Build history of the part. All positions in model axes, mm. A direction names the side the tool comes from. Give positions to 0.01 mm unless a question says otherwise; leave off trailing zeros. Loops run counter-clockwise (first coordinate to the right, second up) from the corner with the lowest first, then second, coordinate; pieces in that order, holes last. Notation, with made-up numbers: M 72.5,10.25 L 122.5,10.25 A23 ccw 122.5,48.25 Z; hole C 80,60 d7. An arc over 180 degrees is marked long. Put each result on its own line as item: value.
Autodesk Inventor part; units mm, degrees
ref_plane "YZ Plane" through (0, 0, 0) normal (1, 0, 0) x (0, 1, 0)
ref_plane "XZ Plane" through (0, 0, 0) normal (0, 1, 0) x (-1, 0, 0)
ref_plane "XY Plane" through (0, 0, 0) normal (0, 0, 1) x (1, 0, 0)
sketch "Sketch1" plane through (0, 0, 0) normal (0, 0, 1) x (1, 0, 0)
  circle A0 centre (0, 0) radius 40
  dimension "d0" = 80
extrude "Extrusion1" add sketch "Sketch1" along normal blind 21.5
sketch "Sketch2" plane through (0, 0, 21.5) normal (0, 0, 1) x (1, 0, 0)
  point P0 (0, 0)
  point P1 (0, 35)
  dimension "d3" = 35
hole "Hole1" at (0, 35, 21.5) direction (0, 0, -1) diameter 4.3 end through all counterbore diameter 10.59 counterbore depth 7
chamfer "Chamfer1" distance 2 distance2 3 2 edges at (-27.6179, -28.9353, 21.5) (28.9353, 27.6179, 21.5) measured on face at (-2.7418, -16.4668, 21.5)
pattern_circular "Circular Pattern1" count 6 over 360 about axis through (0, 0, 0) along (0, 0, 1) of "Hole1"
sketch "Sketch3" plane through (0, 0, 0) normal (0, 0, -1) x (-1, 0, 0)
  circle A0 centre (0, 0) radius 29.1
  dimension "d17" = 58.2
extrude "Extrusion2" cut sketch "Sketch3" against normal through all
ref_plane "Work Plane1" through (0, 0, 10.5) normal (0, 0, -1) x (-1, 0, 0)
sketch "Sketch4" plane through (0, 0, 10.5) normal (0, 0, -1) x (-1, 0, 0)
  circle A0 centre (0, 0) radius 29.5
  circle A1 centre (0, 0) radius 26.5
  dimension "d21" = 53
  dimension "d22" = 59
extrude "Extrusion3" add sketch "Sketch4" against normal blind 3
sketch "Sketch5" plane through (0, 0, 21.5) normal (0, 0, 1) x (1, 0, 0)
  arc A0 (33.6722, 21.5913) -> (1.8625, 39.9566) centre (0, 0) ccw
  line L0 (0, 0) -> (40, 0) construction
  line L1 (21.4926, 23.7527) -> (24.6091, 28.2845)
  line L2 (24.6091, 28.2845) -> (17.6054, 33.101)
  line L3 (17.6054, 33.101) -> (14.4889, 28.5691)
  line L4 (14.4889, 28.5691) -> (21.4926, 23.7527)
  line L5 (21.4926, 23.7527) -> (17.6054, 33.101) construction
  line L6 (24.6091, 28.2845) -> (14.4889, 28.5691) construction
  line L7 (17.002, 26.8409) -> (20.1185, 31.3727)
  line L8 (22.1372, 29.9845) -> (19.0207, 25.4526)
  line L9 (14.8714, 29.1253) -> (17.223, 32.5448)
  line L10 (17.223, 32.5448) -> (19.736, 30.8165)
  line L11 (19.736, 30.8165) -> (17.3845, 27.3971)
  line L12 (17.3845, 27.3971) -> (14.8714, 29.1253)
  line L13 (19.549, 28.4268) -> (16.0472, 30.8351)
  line L14 (17.3845, 27.3971) -> (17.223, 32.5448)
  line L15 (14.8714, 29.1253) -> (19.736, 30.8165)
  line L16 (0, 0) -> (17.3037, 29.9709)
  line L17 (0, 0) -> (19.549, 28.4268)
  dimension "d26" = 8.5
  dimension "d27" = 5.5
  dimension "d29" = 34.5
  dimension "d30" = 3.05
  dimension "d36" = 3
  dimension "d41" = 4.15
  dimension "d42" = 60
extrude "Extrusion4" cut sketch "Sketch5" against normal blind 1.75 contours L4 L17 L13 L7 L2 L8 | L4 L7 L13 L17 | L15 L14 L10 | L7 L13 L15 | L14 L13 L7 | L12 L16 L14 | L14 L13 L3 | L15 L3 L13 | L16 L12 L15
extrude "Extrusion7" cut sketch "Sketch5" against normal through all contours L4 L8 L2 L1
properties part number "Ring_Cover_Top"
Q1. Mould opens along X. For faces 1 (the flat face through (31, 15, 14.5)), 2 (the conical face through (39, 0, 20)), 3 (the cylindrical face through (-8.67, 39.05, 9.12)), 4 (the flat face through (-23, -19, 21.5)) say: pulls with the +X half, pulls with the -X half, needs draft (parallel to the pull), parting line crosses it, or undercut.
Here are the results:
face 1: undercut
face 2: pulls with the +X half
face 3: parting line crosses it
face 4: needs draft
Q2. Probe line 1 (Y direction, x = -26.5, z = 19); line 2 (X direction, y = -17, z = 9.5); line 3 (Y direction, x = -31, z = 12). List the from-to ranges inside material, lowest first. Write a range as from..to.
Here are the results:
line 1: -29.52..-21.18, -13.82..-12.02, 12.02..13.82, 21.18..29.52
line 2: -36.21..-32.4, -28.22..-23.62, 23.62..28.22, 32.4..36.21
line 3: -25.28..-19.54, -15.46..15.46, 19.54..25.28
Q3. Slice it at B-B (y = 0). List the corners of the cut face in (x, z).
Here are the results:
outline: M -40,0 L -29.1,0 L -29.1,10.5 L -26.5,10.5 L -26.5,13.5 L -29.1,13.5 L -29.1,21.5 L -38,21.5 L -40,18.5 Z; M 26.5,10.5 L 29.1,10.5 L 29.1,0 L 40,0 L 40,18.5 L 38,21.5 L 29.1,21.5 L 29.1,13.5 L 26.5,13.5 Z
Q4. Slice it at D-D (z = 7.25). State how many separate pieces and enclosed holes the cut face has, and give its area (3 significant figures).
Here are the results:
separate pieces: 1
enclosed holes: 8
area: 2,260 mm²
Q5. Slice it at C-C (z = 16.75). List the corners of the cut face in (x, y) (1 decimal), and give its area (3 significant figures).
Here are the results:
outline: M -35.5,-18.4 A5.3 cw long -33.7,-21.6 A40 ccw -1.9,-40 A5.3 cw long 1.9,-40 A40 ccw 33.7,-21.6 A5.3 cw long 35.5,-18.4 A40 ccw 35.5,18.4 A5.3 cw long 33.7,21.6 A40 ccw 1.9,40 A5.3 cw long -1.9,40 A40 ccw -33.7,21.6 A5.3 cw long -35.5,18.4 A40 ccw Z; hole C 0,0 d58.2; hole M 19,25.5 L 21.5,23.8 L 24.6,28.3 L 22.1,30 Z
area: 1,830 mm²
Q6. Drop flat-ended pins along their axis: pin 1 Ø5 at (y, z) = (19, 2.5) entering from +X; pin 2 Ø3 at (x, y) = (-1, 35) entering from +Z; pin 3 Ø5 at (x, z) = (-22.5, 15) entering from +Y. Give the stop position or say it passes through.
Here are the results:
pin 1: x = 36.44
pin 2: z = 14.5
pin 3: y = 34.64
Q7. Tool access for faces 5 (the flat face through (-28, 16, 14.5)), 6 (the conical face through (19.62, -33.464, 20.312)), 7 (the flat face through (23.03, 25.99, 10.9)): list every direction of +Z, -Z, +X, -X, +Y, -Y with a clear straight run to the whole face (end or side of a thin tool).
Here are the results:
face 5: +Z
face 6: +Z, +X, -Y
face 7: +Z, -Z
Q8. Slice it at A-A (x = 0). List the corners of the cut face in (y, z) (3 decimals), and give its area (3 significant figures).
Here are the results:
outline: M -40,0 L -37.15,0 L -37.15,14.5 L -40,14.5 Z; M -32.85,0 L -29.1,0 L -29.1,10.5 L -26.5,10.5 L -26.5,13.5 L -29.1,13.5 L -29.1,21.5 L -29.705,21.5 L -29.705,14.5 L -32.85,14.5 Z; M 26.5,10.5 L 29.1,10.5 L 29.1,0 L 32.85,0 L 32.85,14.5 L 29.705,14.5 L 29.705,21.5 L 29.1,21.5 L 29.1,13.5 L 26.5,13.5 Z; M 37.15,0 L 40,0 L 40,14.5 L 37.15,14.5 Z
area: 215 mm²
